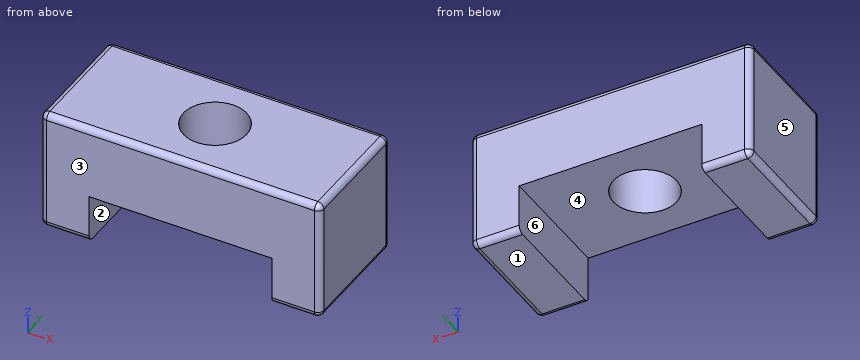
```python
from build123d import *

# Parameters (mm, degrees)
F1_DEPTH = 20
F2_R     = 5.2
F3_DEPTH = 25
F4_R     = 1


with BuildPart() as f1:
    # F0 (on Front) → F1 (new body)
    with BuildSketch(Plane.XZ):
        with BuildLine():
            Line((22, 10), (-22, 10))
            ThreePointArc((-22, 10), (-22.7071067812, 9.7071067812), (-23, 9))
            Line((-23, 9), (-23, -9))
            ThreePointArc((-23, -9), (-22.7071067812, -9.7071067812), (-22, -10))
            Line((-22, -10), (-15, -10))
            Line((-15, -10), (-15, -2))
            Line((-15, -2), (15, -2))
            Line((15, -2), (15, -10))
            Line((15, -10), (22, -10))
            ThreePointArc((22, -10), (22.7071067812, -9.7071067812), (23, -9))
            Line((23, -9), (23, 9))
            ThreePointArc((23, 9), (22.7071067812, 9.7071067812), (22, 10))
        make_face()
    extrude(amount=F1_DEPTH)

    # F2 (on face) → F3 (cut)
    with BuildSketch(Plane.XY.offset(10)):
        with Locations((0, -10)):
            Circle(F2_R)
    extrude(amount=-F3_DEPTH, mode=Mode.SUBTRACT)

    # F4
    f4_edges = [f1.edges().sort_by_distance(p)[0] for p in [
        (0, -20, 10),
        (23, -20, 0),
        (0, 0, 10),
        (23, 0, 0),
    ]]
    fillet(f4_edges, radius=F4_R)


solid = f1.part
```
Read the model definition and answer for the solid it produces. Units are mm, in the model's axes. Face numbers are marked on the shaded views. A direction names the side the tool comes from. Give positions to 0.01 mm unless a question says otherwise; leave off trailing zeros. Write each loop counter-clockwise with the first axis right and the second up, starting at its lowest first coordinate (ties: lowest second). Pieces come first, ordered by that corner, then holes. Notation, with made-up numbers: (-24.75, -13) -> (9.25, -13) arc R8 cw to (9.25, -8) -> close; hole circle Ø10 at (30.25, 14.25). An arc over 180 degrees is marked (long way). Answer in a Markdown table with one row per item.
1) Straight lines are drawn through the part: line 1 (Y direction, x = 0, z = 5.25); line 2 (X direction, y = -5.25, z = -5.25); line 3 (X direction, y = -9.75, z = 8). For each, find the intervals that lie inside material, in ascending order. Write a range as [from, to].
Results list:
| item | result |
|---|---|
| line 1 | [-20, -15.2], [-4.8, 0] |
| line 2 | [-23, -15], [15, 23] |
| line 3 | [-23, -5.19], [5.19, 23] |
2) Section B-B on x = 0 is taken. Give the vertices of the cut face in (y, z), plus the area to 3 significant figures.
Results list:
| item | result |
|---|---|
| outline | (-20, -2) -> (-15.2, -2) -> (-15.2, 10) -> (-19, 10) arc R1 ccw to (-20, 9) -> close; (-4.8, -2) -> (0, -2) -> (0, 9) arc R1 ccw to (-1, 10) -> (-4.8, 10) -> close |
| area | 115 mm^2 |
3) A tool of negligible diameter and unlimited length cuts with its end or side. For the marked faces 1 and 2, from which of +Z, -Z, +X, -X, +Y, -Y can it reach the whole face along a straight path? Write none if from no direction.
Results list:
| item | result |
|---|---|
| face 1 | -Z, +X, -X, +Y, -Y |
| face 2 | -Z, +Y, -Y |
4) Section D-D on y = -2.25 is taken. Give the vertices of the cut face in (x, z).
Results list:
| item | result |
|---|---|
| outline | (-23, -9) arc R1 ccw to (-22, -10) -> (-15, -10) -> (-15, -2) -> (15, -2) -> (15, -10) -> (22, -10) arc R1 ccw to (23, -9) -> (23, 9) arc R1 ccw to (22, 10) -> (-22, 10) arc R1 ccw to (-23, 9) -> close |
5) This flat-tipped pin is pushed along its axis until it touches: pin 1 Ø10 at (x, y) = (-5, -11) entering from -Z. Where does it stop, or does it pass through?
Results list:
| item | result |
|---|---|
| pin 1 | z = -2 |
6) Determine the mould class of the marked faces 3, 4, 5 and 6 for opening direction X: released by +X, released by -X, zero draft, split by the parting line, or undercut.
Results list:
| item | result |
|---|---|
| face 3 | zero draft |
| face 4 | undercut |
| face 5 | released by -X |
| face 6 | undercut |
7) Section C-C on z = 6.75 is taken. Give the vertices of the cut face in (x, y), plus the area to 3 significant figures.
Results list:
| item | result |
|---|---|
| outline | (-23, -19) arc R1 ccw to (-22, -20) -> (22, -20) arc R1 ccw to (23, -19) -> (23, -1) arc R1 ccw to (22, 0) -> (-22, 0) arc R1 ccw to (-23, -1) -> close; hole circle Ø10.4 at (0, -10) |
| area | 834 mm^2 |
8) Section A-A on y = -10 is taken. Give the vertices of the cut face in (x, z).
Results list:
| item | result |
|---|---|
| outline | (-23, -9) arc R1 ccw to (-22, -10) -> (-15, -10) -> (-15, -2) -> (-5.2, -2) -> (-5.2, 10) -> (-22, 10) arc R1 ccw to (-23, 9) -> close; (5.2, -2) -> (15, -2) -> (15, -10) -> (22, -10) arc R1 ccw to (23, -9) -> (23, 9) arc R1 ccw to (22, 10) -> (5.2, 10) -> close |
